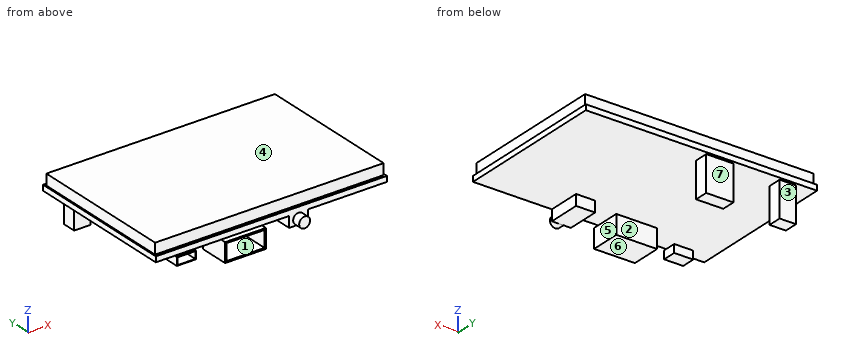
from build123d import *

# Parameters (mm, degrees)
ESQUISSE1_W        = 85
ESQUISSE1_H        = 56
BOSS_EXTRU_1_DEPTH = 2
ESQUISSE2_W        = 84
ESQUISSE2_H        = 54
BOSS_EXTRU_2_DEPTH = 4
ESQUISSE3_W        = 6
ESQUISSE3_H        = 5
ESQUISSE3_W_2      = 10
BOSS_EXTRU_3_DEPTH = 13
ESQUISSE4_W        = 15
ESQUISSE4_H        = 11
BOSS_EXTRU_4_DEPTH = 7
COQUE1_T           = -0.5
ESQUISSE5_W        = 7
ESQUISSE5_H        = 5
BOSS_EXTRU_5_DEPTH = 3
COQUE2_T           = -0.2
ESQUISSE6_W        = 7
ESQUISSE6_H        = 12
BOSS_EXTRU_6_DEPTH = 4
ESQUISSE7_R        = 2
BOSS_EXTRU_7_DEPTH = 3


with BuildPart() as part:
    # Esquisse1 → Boss.-Extru.1 (new body)
    with BuildSketch(Plane.XY):
        Rectangle(ESQUISSE1_W, ESQUISSE1_H)
    extrude(amount=BOSS_EXTRU_1_DEPTH)

    # Esquisse2 → Boss.-Extru.2 (add)
    with BuildSketch(Plane.XY.offset(2)):
        Rectangle(ESQUISSE2_W, ESQUISSE2_H)
    extrude(amount=BOSS_EXTRU_2_DEPTH)

    # Esquisse3 → Boss.-Extru.3 (add)
    with BuildSketch(Plane(origin=(0, 0, 0), x_dir=(-1, 0, 0), z_dir=(0, 0, -1))):
        with Locations((32.5, 24.5)):
            Rectangle(ESQUISSE3_W, ESQUISSE3_H)
        with Locations((7.5, 24.5)):
            Rectangle(ESQUISSE3_W_2, ESQUISSE3_H)
    extrude(amount=BOSS_EXTRU_3_DEPTH)

    # Esquisse4 → Boss.-Extru.4 (add)
    with BuildSketch(Plane(origin=(0, 0, 0), x_dir=(-1, 0, 0), z_dir=(0, 0, -1))):
        with Locations((11, -24.5)):
            Rectangle(ESQUISSE4_W, ESQUISSE4_H)
    extrude(amount=BOSS_EXTRU_4_DEPTH)

    # Coque1
    coque1_openings = [part.faces().sort_by_distance(p)[0] for p in [
        (-11, -30, -3.5),
    ]]
    offset(amount=COQUE1_T, openings=coque1_openings, kind=Kind.INTERSECTION)

    # Esquisse5 → Boss.-Extru.5 (add)
    with BuildSketch(Plane(origin=(0, 0, 0), x_dir=(-1, 0, 0), z_dir=(0, 0, -1))):
        with Locations((32, -26.5)):
            Rectangle(ESQUISSE5_W, ESQUISSE5_H)
    extrude(amount=BOSS_EXTRU_5_DEPTH)

    # Coque2
    coque2_openings = [part.faces().sort_by_distance(p)[0] for p in [
        (-32, -29, -1.5),
    ]]
    offset(amount=COQUE2_T, openings=coque2_openings, kind=Kind.INTERSECTION)

    # Esquisse6 → Boss.-Extru.6 (add)
    with BuildSketch(Plane(origin=(0, 0, 0), x_dir=(-1, 0, 0), z_dir=(0, 0, -1))):
        with Locations((-10, -22)):
            Rectangle(ESQUISSE6_W, ESQUISSE6_H)
    extrude(amount=BOSS_EXTRU_6_DEPTH)

    # Esquisse7 → Boss.-Extru.7 (add)
    with BuildSketch(Plane.XZ.offset(28)):
        with Locations((10, -2)):
            Circle(ESQUISSE7_R)
    extrude(amount=BOSS_EXTRU_7_DEPTH)


solid = part.part
The model under review builds one solid part; all positions refer to its coordinate system, in mm. Face numbers are marked on the shaded views. A direction names the side the tool comes from. Round coordinates to 2 decimals unless told otherwise and drop trailing zeros. Loops run counter-clockwise (first coordinate to the right, second up) from the corner with the lowest first, then second, coordinate; pieces in that order, holes last. Notation, with made-up numbers: (47.5, 14.5) -> (101.5, 14.5) arc R28 cw to (101.5, 50.5) -> close; hole circle Ø10 at (16.5, -21.5). An arc over 180 degrees is marked (long way). Write item = value, one per line. Start each with the question number.
Item 1: Take a section at C-C on z = 4. Give the boundary of the cut face in (x, y), plus the area to 3 significant figures.
Item 2: Mouldability with a two-part tool opening along Y and no side actions: class the marked faces 1, 2 and 3 as released by +Y, released by -Y, zero draft, split by the parting line, or undercut.
Item 3: Take a section at A-A on x = 25.5. Count the separate pieces of the cut face and the enclosed holes in it, plus the area to 3 significant figures.
Item 4: To check wall thickness, follow L1, parallel to X at y = 5.5, z = 1.75. State the ranges of the line that lie inside material, in increasing order.
Item 5: Insertion check: pin 1 (1.5 mm diameter, centred on x = -28.5, z = -2, fed in from +Y); pin 2 (4.5 mm diameter, centred on x = -13, z = 5, fed in from -Y); pin 3 (4.5 mm diameter, centred on y = 24.5, z = -8, fed in from -X); pin 4 (6 mm diameter, centred on y = 17, z = -7.5, fed in from +X). Each pin has a flat end and moves straight along its axis. Give the tip position at first contact, or say it passes through.
Item 6: For the marked faces 4, 5, 6 and 7, list the 3-axis set-ups (+Z, -Z, +X, -X, +Y, -Y) from which the entire face can be reached by the end or side of a thin tool; tool diameter is ignored.
Result:
q1.outline = (-42, -27) -> (42, -27) -> (42, 27) -> (-42, 27) -> close; (-41.7, -26.7) -> (41.7, -26.7) -> (41.7, 26.7) -> (-41.7, 26.7) -> close; hole (-41.8, -26.8) -> (41.8, -26.8) -> (41.8, 26.8) -> (-41.8, 26.8) -> close; hole (-41.5, -26.5) -> (41.5, -26.5) -> (41.5, 26.5) -> (-41.5, 26.5) -> close
q1.area = 110 mm²
q2.face_1 = zero draft
q2.face_2 = undercut
q2.face_3 = released by +Y
q3.separate_pieces = 2
q3.enclosed_holes = 2
q3.area = 48.8 mm²
q4.L1 = -42.5 to -42.3, -41.7 to -41.5, 41.5 to 41.7, 42.3 to 42.5
q5.pin_1 = -24
q5.pin_2 = -27
q5.pin_3 = -35.5
q5.pin_4 = through
q6.face_4 = +Z, +X, -X, +Y, -Y
q6.face_5 = -Z, -Y
q6.face_6 = -Z, +X, -X, -Y
q6.face_7 = -Z, +X, -X, +Y
